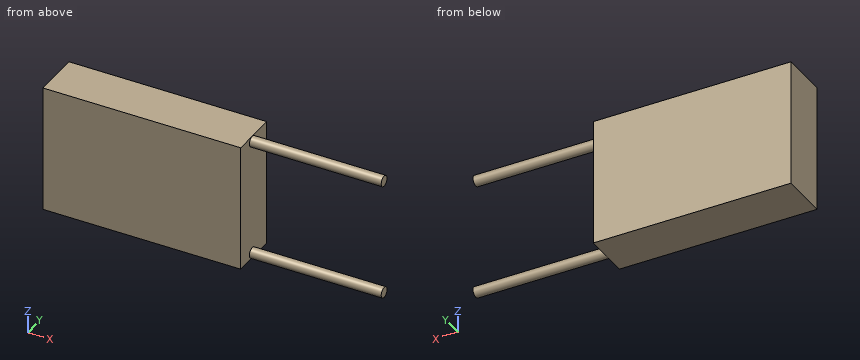
```python
from build123d import *

# Parameters (mm, degrees)
SKETCH2_W           = 37.5
SKETCH2_H           = 24.2
BOSS_EXTRUDE1_DEPTH = 9
SKETCH3_R           = 1
BOSS_EXTRUDE2_DEPTH = 25


with BuildPart() as part:
    # Sketch2 → Boss-Extrude1 (new body)
    with BuildSketch(Plane(origin=(0, 0, 0), x_dir=(1, 0, 0), z_dir=(0, 1, 0))):
        Rectangle(SKETCH2_W, SKETCH2_H)
    extrude(amount=BOSS_EXTRUDE1_DEPTH)

    # Sketch3 → Boss-Extrude2 (add)
    with BuildSketch(Plane(origin=(18.75, 0, 0), x_dir=(0, 0, -1), z_dir=(1, 0, 0))):
        with Locations(Location((-11.1, 4, 0), (0, 0, 180))):
            Circle(SKETCH3_R)
    boss_extrude2 = extrude(amount=BOSS_EXTRUDE2_DEPTH)

    # Mirror1: Boss-Extrude2 across plane
    add(boss_extrude2.mirror(Plane.XY))


solid = part.part
```
Work out the finished part from the listing and answer in its coordinate system (mm). Coordinates: 2 decimals unless noted, no trailing zeros. Loops run counter-clockwise (first coordinate to the right, second up) from the corner with the lowest first, then second, coordinate; pieces in that order, holes last. Notation, with made-up numbers: M 82.5,0.5 L 137.5,0.5 A11 cw 137.5,8.5 Z; hole C -16.5,-31 d3. An arc over 180 degrees is marked long. Use CSV: the item, a comma, the result in double quotes. Start each with the question number.
(1) Given pin 1 Ø1 at (x, y) = (19, 2) entering from +Z; pin 2 Ø5 at (y, z) = (7, 7) entering from +X, each flat-ended and moving along its own axis, determine where each tip first touches the part or whether it passes through.
(2) Find section D-D, the plane z = 1.25. Give the vertices of the cut face in (x, y).
(3) Find section A-A, the plane z = 11.1. Give the vertices of the cut face in (x, y), then the cut area to 4 significant figures.
(4) Consider line 1 (X direction, y = 2.75, z = 2.5); line 2 (Z direction, x = 25, y = 4.75); line 3 (Y direction, x = 29, z = 10.75). Determine where each line is inside the solid, lowest interval first.
(5) Find section B-B, the plane x = 31.5. Give the vertices of the cut face in (y, z), then the cut area to 3 significant figures.
(6) Find section C-C, the plane y = 1.25. Give the vertices of the cut face in (x, z).
Recorded:
1,pin 1,"stops at z = 12.1"
1,pin 2,"stops at x = 18.75"
2,outline,"M -18.75,0 L 18.75,0 L 18.75,9 L -18.75,9 Z"
3,outline,"M -18.75,0 L 18.75,0 L 18.75,3 L 43.75,3 L 43.75,5 L 18.75,5 L 18.75,9 L -18.75,9 Z"
3,area,"387.5 mm^2"
4,line 1,"x = -18.75 to 18.75"
4,line 2,"z = -11.76 to -10.44, 10.44 to 11.76"
4,line 3,"y = 3.06 to 4.94"
5,outline,"C 4,-11.1 d2; C 4,11.1 d2"
5,area,"6.28 mm^2"
6,outline,"M -18.75,-12.1 L 18.75,-12.1 L 18.75,12.1 L -18.75,12.1 Z"
